Solid Edge part; units mm, degrees
sketch "Sketch1" plane through (0, 0, 0) normal (0, 0, 1) x (1, 0, 0)
  line L0 (0, -7.2579) -> (56, -7.2579)
  line L1 (56, -7.2579) -> (56, 17.2421)
  line L2 (56, 17.2421) -> (0, 17.2421)
  line L3 (0, 17.2421) -> (0, -7.2579)
extrude "Protrusion1" add sketch "Sketch1" along normal blind 11
hole "Hole_1" at (52.5, 12.7421, 11) direction (0, 0, -1) diameter 3.3 end through all
hole "Hole1" at (3.5, 12.7421, 11) direction (0, 0, -1) diameter 3.3 end through all
sketch "Sketch2" plane through (28, 4.9921, 11) normal (0, 0, 1) x (1, 0, 0)
  line L0 (-21, 4.25) -> (21, 4.25)
  arc A0 (22, 5.25) -> (21, 4.25) centre (21, 5.25) cw
  line L1 (22, 5.25) -> (22, 12.25)
  line L2 (22, 12.25) -> (-22, 12.25)
  line L3 (-22, 12.25) -> (-22, 5.25)
  arc A1 (-22, 5.25) -> (-21, 4.25) centre (-21, 5.25) ccw
extrude "ExtrudedCutout_1" cut sketch "Sketch2" against normal blind 1
sketch "Sketch3" plane through (28, 4.9921, 11) normal (0, 0, 1) x (1, 0, 0)
  line L0 (-28, 12.25) -> (28, 12.25)
  line L1 (28, 12.25) -> (28, 11.25)
  line L2 (28, 11.25) -> (-28, 11.25)
  line L3 (-28, 11.25) -> (-28, 12.25)
extrude "Cutout1" cut sketch "Sketch3" against normal through all
properties material "Aluminum, 6061-T6"
Build history of the part. All positions in model axes, mm. A direction names the side the tool comes from. Give positions to 0.01 mm unless a question says otherwise; leave off trailing zeros. Loops run counter-clockwise (first coordinate to the right, second up) from the corner with the lowest first, then second, coordinate; pieces in that order, holes last.
1) Band-saw the part on A-A on x = 3.5. List the corners of the cut face in (y, z), then the cut area to 3 significant figures.
Values follow:
outline: (-7.26, 0) - (11.09, 0) - (11.09, 11) - (-7.26, 11) - close; (14.39, 0) - (16.24, 0) - (16.24, 11) - (14.39, 11) - close
area: 222 mm2
2) Probe line 1 along X through (y, z) = (12.75, 4); line 2 along Y through (x, z) = (52.5, 3.75); line 3 along X through (y, z) = (12, 1). List the from-to ranges inside material, lowest first.
Values follow:
line 1: x = 0 to 1.85, 5.15 to 50.85, 54.15 to 56
line 2: y = -7.26 to 11.09, 14.39 to 16.24
line 3: x = 0 to 2.03, 4.97 to 51.03, 53.97 to 56
3) Band-saw the part on B-B on x = 32. List the corners of the cut face in (y, z).
Values follow:
outline: (-7.26, 0) - (16.24, 0) - (16.24, 10) - (9.24, 10) - (9.24, 11) - (-7.26, 11) - close
4) Band-saw the part on C-C on x = 53. List the corners of the cut face in (y, z).
Values follow:
outline: (-7.26, 0) - (11.17, 0) - (11.17, 11) - (-7.26, 11) - close; (14.31, 0) - (16.24, 0) - (16.24, 11) - (14.31, 11) - close
5) 3-axis set-ups, long thin cutter, end or side, ignore diameter. For faces 1 (the face through (28, -7.258, 5)), 2 (the face through (6, 13.3, 10.5)): which of +Z, -Z, +X, -X, +Y, -Y reach the whole face in a straight line?
Values follow:
face 1: +Z, -Z, +X, -X, -Y
face 2: +Z, +Y
